Design review of the part built by this model. Coordinates are the model's own, in mm. Face numbers are marked on the shaded views. A direction names the side the tool comes from. Round coordinates to 2 decimals unless told otherwise and drop trailing zeros. Write each loop counter-clockwise with the first axis right and the second up, starting at its lowest first coordinate (ties: lowest second). Pieces come first, ordered by that corner, then holes. Notation, with made-up numbers: (1.25, 78.25) -> (55.25, 78.25) arc R14 ccw to (55.25, 103.25) -> close; hole circle Ø8 at (61.5, 66). An arc over 180 degrees is marked (long way). One line per question, with ' | ' between items. Start each with the question number.
1) For the marked faces 1 and 2, list the 3-axis set-ups (+Z, -Z, +X, -X, +Y, -Y) from which the entire face can be reached by the end or side of a thin tool; tool diameter is ignored.
2) Consider section D-D (y = 0). Give the boundary of the cut face in (x, z).
3) Consider section C-C (x = -34). Give the boundary of the cut face in (y, z), then the cut area to 3 significant figures.
4) Insertion check: pin 1 Ø6.5 at (x, y) = (-34, 0) entering from +Z (3 decimals); pin 2 Ø2 at (y, z) = (6, 56) entering from +X; pin 3 Ø8 at (x, z) = (-14, 104.5) entering from -Y; pin 4 Ø4 at (x, z) = (-2, 89) entering from +Y. Each pin has a flat end and moves straight along its axis. Give the tip position at first contact, or say it passes through.
5) Consider section A-A (x = 0). Give the boundary of the cut face in (y, z), then the cut area to 3 significant figures.
6) Consider section B-B (y = -35). Give the boundary of the cut face in (x, z), then the cut area to 3 significant figures.
7) For probe 1 along Y at (x, z) = (34, 1.3); probe 2 along Y at (x, z) = (0, 0.85); probe 3 along Z at (x, y) = (39.5, -33), list the stretches that pass through material, from the lowest coordinate up.
```python
from build123d import *

# Parameters (mm, degrees)
F0_R     = 5.5
F0_R_2   = 12
F1_DEPTH = 4
F2_R     = 12
F3_DEPTH = 130
F4_R     = 4


with BuildPart() as f1:
    # F0 (on Top) → F1 (new body)
    with BuildSketch(Plane.XY):
        Polygon((50, 50), (0, 50), (-50, 50), (-50, -70), (0, -70), (50, -70), align=None)
        with Locations((-34, -54)):
            Circle(F0_R, mode=Mode.SUBTRACT)
        with Locations((34, -54)):
            Circle(F0_R, mode=Mode.SUBTRACT)
        with Locations((0, -35)):
            Circle(F0_R, mode=Mode.SUBTRACT)
        with Locations((-34, 0)):
            Circle(F0_R, mode=Mode.SUBTRACT)
        Circle(F0_R_2, mode=Mode.SUBTRACT)
        with Locations((34, 0)):
            Circle(F0_R, mode=Mode.SUBTRACT)
    extrude(amount=F1_DEPTH)

    # F2 (on face) → F3 (join)
    with BuildSketch(Plane(origin=(0, 0, 0), x_dir=(1, 0, 0), z_dir=(0, 0, -1))):
        Circle(F2_R)
    extrude(amount=-F3_DEPTH)

    # F4
    f4_edges = [f1.edges().sort_by_distance(p)[0] for p in [
        (-12, 0, 4),
    ]]
    fillet(f4_edges, radius=F4_R)


solid = f1.part
```
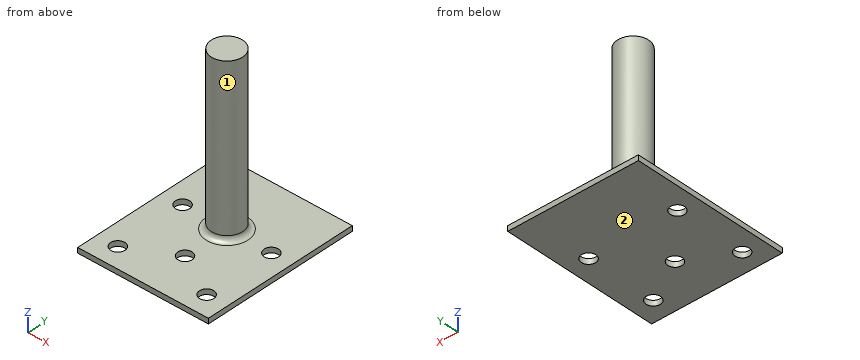
From the geometry:
1) face 1: +Z | face 2: -Z, +X, -X, +Y, -Y
2) outline: (-50, 0) -> (-39.5, 0) -> (-39.5, 4) -> (-50, 4) -> close; (-28.5, 0) -> (28.5, 0) -> (28.5, 4) -> (16, 4) arc R4 cw to (12, 8) -> (12, 130) -> (-12, 130) -> (-12, 8) arc R4 cw to (-16, 4) -> (-28.5, 4) -> close; (39.5, 0) -> (50, 0) -> (50, 4) -> (39.5, 4) -> close
3) outline: (-70, 0) -> (-59.5, 0) -> (-59.5, 4) -> (-70, 4) -> close; (-48.5, 0) -> (-5.5, 0) -> (-5.5, 4) -> (-48.5, 4) -> close; (5.5, 0) -> (50, 0) -> (50, 4) -> (5.5, 4) -> close | area: 392 mm2
4) pin 1: passes through | pin 2: stops at x = 10.91 | pin 3: stops at y = -6.63 | pin 4: stops at y = 12
5) outline: (-70, 0) -> (-40.5, 0) -> (-40.5, 4) -> (-70, 4) -> close; (-29.5, 0) -> (50, 0) -> (50, 4) -> (16, 4) arc R4 cw to (12, 8) -> (12, 130) -> (-12, 130) -> (-12, 8) arc R4 cw to (-16, 4) -> (-29.5, 4) -> close | area: 3,470 mm2
6) outline: (-50, 0) -> (-5.5, 0) -> (-5.5, 4) -> (-50, 4) -> close; (5.5, 0) -> (50, 0) -> (50, 4) -> (5.5, 4) -> close | area: 356 mm2
7) probe 1: y = -70 to -59.5, -48.5 to -5.5, 5.5 to 50 | probe 2: y = -70 to -40.5, -29.5 to 50 | probe 3: z = 0 to 4
